Can you work these out from the model? Positions are in its coordinate system, mm. A direction names the side the tool comes from. Give positions to 0.01 mm unless a question says otherwise; leave off trailing zeros. Order: outer loops, then holes, each group sorted by start corner. A loop starts at its lowest first (then second) coordinate and runs counter-clockwise, first axis right, second up. Notation, with made-up numbers: (32.25, 40.25) - (83.25, 40.25) arc R19 ccw to (83.25, 68.25) - close; hole circle Ø9 at (68.5, 79.5). An arc over 180 degrees is marked (long way). Return JSON: item names as keys, results as strings.
```python
from build123d import *

# Parameters (mm, degrees)
SKETCH1_W               = 95.25
SKETCH1_H               = 8.466666667
BOSS_EXTRUDE1_DEPTH     = 38.1
SKETCH2_W               = 6.35
SKETCH2_H               = 127
BOSS_EXTRUDE2_DEPTH     = 38.1
SKETCH3_W               = 88.9
SKETCH3_H               = 8.466666667
BOSS_EXTRUDE3_DEPTH     = 38.1
SKETCH4_R               = 11
CUT_EXTRUDE1_DEPTH      = 149.412147835
SKETCH5_R               = 2.15265
CUT_EXTRUDE2_DEPTH      = 149.412147835
FILLET1_R               = 7.62
BOSS_EXTRUDE4_DEPTH     = 38.1
CUT_EXTRUDE8_REACH      = 172.773
CUT_EXTRUDE8_END_RADIUS = 38.1
FILLET2_R               = 11.688947
FILLET3_R               = 11.688947
FILLET4_R               = 6.35
BOSS_EXTRUDE7_START     = -38.1
BOSS_EXTRUDE7_DEPTH     = 38.1
CUT_EXTRUDE12_DEPTH     = 157.640484095


with BuildPart() as part:
    # Sketch1 → Boss-Extrude1 (new body)
    with BuildSketch(Plane(origin=(0, 0, 0), x_dir=(1, 0, 0), z_dir=(0, 1, 0))):
        with Locations((19.05, 13.758333334)):
            Rectangle(SKETCH1_W, SKETCH1_H)
    extrude(amount=BOSS_EXTRUDE1_DEPTH)

    # Sketch2 → Boss-Extrude2 (add)
    with BuildSketch(Plane(origin=(0, 38.1, 0), x_dir=(1, 0, 0), z_dir=(0, 1, 0))):
        with Locations((63.5, 73.025)):
            Rectangle(SKETCH2_W, SKETCH2_H)
    extrude(amount=-BOSS_EXTRUDE2_DEPTH)

    # Sketch3 → Boss-Extrude3 (add)
    with BuildSketch(Plane(origin=(0, 38.1, 0), x_dir=(1, 0, 0), z_dir=(0, 1, 0))):
        with Locations((15.875, 132.291666667)):
            Rectangle(SKETCH3_W, SKETCH3_H)
    extrude(amount=-BOSS_EXTRUDE3_DEPTH)

    # Sketch4 → Cut-Extrude1 (cut, through all)
    with BuildSketch(Plane(origin=(0, 0, -136.525), x_dir=(-1, 0, 0), z_dir=(0, 0, -1))):
        with Locations((-31.75, 19.05)):
            Circle(SKETCH4_R)
    extrude(amount=-CUT_EXTRUDE1_DEPTH, mode=Mode.SUBTRACT)

    # Sketch5 → Cut-Extrude2 (cut, through all)
    with BuildSketch(Plane(origin=(0, 0, -136.525), x_dir=(-1, 0, 0), z_dir=(0, 0, -1))):
        with Locations((-18.877667779, 26.704865736)):
            Circle(SKETCH5_R)
        with Locations((-19.228536904, 10.833743663)):
            Circle(SKETCH5_R)
        with Locations((-44.622332221, 11.395134264)):
            Circle(SKETCH5_R)
        with Locations((-44.271463096, 27.266256337)):
            Circle(SKETCH5_R)
    extrude(amount=-CUT_EXTRUDE2_DEPTH, mode=Mode.SUBTRACT)

    # Fillet1
    fillet1_edges = [part.edges().sort_by_distance(p)[0] for p in [
        (66.675, 19.05, -136.525),
        (66.675, 19.05, -9.525),
    ]]
    fillet(fillet1_edges, radius=FILLET1_R)

    # Sketch10 → Boss-Extrude4 (add)
    with BuildSketch(Plane(origin=(0, 38.1, 0), x_dir=(1, 0, 0), z_dir=(0, 1, 0))):
        with BuildLine():
            Line((-28.575, 17.991666667), (-28.575, 9.525))
            Line((-28.575, 9.525), (-34.925, 9.525))
            Line((-34.925, 9.525), (-34.925, 25.781))
            Line((-34.925, 25.781), (-5.996027965, 57.15))
            ThreePointArc((-5.996027965, 57.15), (-2.531188929, 73.025), (-5.996027965, 88.9))
            Line((-5.996027965, 88.9), (-34.925, 120.269))
            Line((-34.925, 120.269), (-34.925, 136.525))
            Line((-34.925, 136.525), (-28.575, 136.525))
            Line((-28.575, 136.525), (-28.575, 123.825))
            Line((-28.575, 123.825), (-10.494392478, 104.219375))
            ThreePointArc((-10.494392478, 104.219375), (2.742945437, 73.025), (-10.494392478, 41.830625))
            Line((-10.494392478, 41.830625), (-28.575, 22.225))
            Line((-28.575, 22.225), (-28.575, 17.991666667))
        make_face()
    extrude(amount=-BOSS_EXTRUDE4_DEPTH)

    # Cut-Extrude8: up to this cylinder (the profile starts outside it)
    cut_extrude8_end = Plane(origin=(-40.631188929, 4.042536, -73.025), z_dir=(0, 1, 0)) * Cylinder(CUT_EXTRUDE8_END_RADIUS, 422.746, mode=Mode.PRIVATE)
    # Sketch12 → Cut-Extrude8 (cut, up to the surface)
    with BuildSketch(Plane.ZY.offset(-60.325), mode=Mode.PRIVATE) as cut_extrude8_sk1:
        with BuildLine():
            Line((-82.55, 0), (-63.5, 0))
            ThreePointArc((-63.5, 0), (-73.025, 9.525), (-82.55, 0))
        make_face()
    cut_extrude8_tool1 = extrude(cut_extrude8_sk1.sketch, amount=CUT_EXTRUDE8_REACH, mode=Mode.PRIVATE) - cut_extrude8_end
    add(cut_extrude8_tool1.solids().sort_by_distance((60.325, 4.042536, -73.025))[0], mode=Mode.SUBTRACT)

    # Fillet2
    fillet2_edges = [part.edges().sort_by_distance(p)[0] for p in [
        (-34.925, 19.05, -136.525),
        (-34.925, 19.05, -120.269),
    ]]
    fillet(fillet2_edges, radius=FILLET2_R - 0.0001)  # a hair under: the kernel refuses the full size

    # Fillet3
    fillet3_edges = [part.edges().sort_by_distance(p)[0] for p in [
        (-34.925, 19.05, -25.781),
        (-34.925, 19.05, -9.525),
    ]]
    fillet(fillet3_edges, radius=FILLET3_R - 0.0001)  # a hair under: the kernel refuses the full size

    # Fillet4
    fillet4_edges = [part.edges().sort_by_distance(p)[0] for p in [
        (60.325, 19.05, -17.991666667),
        (60.325, 19.05, -128.058333333),
    ]]
    fillet(fillet4_edges, radius=FILLET4_R)

    # Sketch15 → Boss-Extrude7 (add)
    with BuildSketch(Plane(origin=(0, 38.1, 0), x_dir=(1, 0, 0), z_dir=(0, 1, 0)).offset(BOSS_EXTRUDE7_START)):
        with BuildLine():
            Line((-27.874453006, 23.470813729), (-27.581873113, 23.301892649))
            Line((-27.581873113, 23.301892649), (-25.057662874, 26.039008606))
            ThreePointArc((-25.057662874, 26.039008606), (-34.066608211, 16.896224406), (-21.277878592, 17.991666667))
            Line((-21.277878592, 17.991666667), (-24.699453006, 17.991666667))
            Line((-24.699453006, 17.991666667), (-24.699453006, 17.971552415))
            Line((-24.699453006, 17.971552415), (-27.874453006, 16.13846531))
            Line((-27.874453006, 16.13846531), (-31.049453006, 17.971552415))
            Line((-31.049453006, 17.971552415), (-31.049453006, 21.637726624))
            Line((-31.049453006, 21.637726624), (-27.874453006, 23.470813729))
        make_face()
        with BuildLine():
            Line((-27.581873113, 23.301892649), (-24.699453006, 21.637726624))
            Line((-24.699453006, 21.637726624), (-24.699453006, 17.991666667))
            Line((-24.699453006, 17.991666667), (-21.277878592, 17.991666667))
            ThreePointArc((-21.277878592, 17.991666667), (-21.094704511, 18.889940166), (-21.033278796, 19.804639519))
            ThreePointArc((-21.033278796, 19.804639519), (-22.126765794, 23.514862731), (-25.057662874, 26.039008606))
            Line((-25.057662874, 26.039008606), (-27.581873113, 23.301892649))
        make_face()
        with BuildLine():
            ThreePointArc((60.325, 26.609850645), (54.403432166, 24.225341495), (53.027878592, 17.991666667))
            Line((53.027878592, 17.991666667), (53.975, 17.991666667))
            ThreePointArc((53.975, 17.991666667), (55.237426297, 18.118421545), (56.449453006, 18.493625771))
            Line((56.449453006, 18.493625771), (56.449453006, 21.637726624))
            Line((56.449453006, 21.637726624), (59.624453006, 23.470813729))
            Line((59.624453006, 23.470813729), (60.208975135, 23.13333972))
            ThreePointArc((60.208975135, 23.13333972), (60.295927231, 23.734724375), (60.325, 24.341666667))
            Line((60.325, 24.341666667), (60.325, 26.609850645))
        make_face()
        with BuildLine():
            Line((53.975, 17.991666667), (53.027878592, 17.991666667))
            ThreePointArc((53.027878592, 17.991666667), (60.539152358, 13.024891024), (66.465627215, 19.804639519))
            ThreePointArc((66.465627215, 19.804639519), (64.703538976, 24.387711662), (60.325, 26.609850645))
            Line((60.325, 26.609850645), (60.325, 24.341666667))
            ThreePointArc((60.325, 24.341666667), (60.295927231, 23.734724375), (60.208975135, 23.13333972))
            Line((60.208975135, 23.13333972), (62.799453006, 21.637726624))
            Line((62.799453006, 21.637726624), (62.799453006, 17.971552415))
            Line((62.799453006, 17.971552415), (59.624453006, 16.13846531))
            Line((59.624453006, 16.13846531), (56.449453006, 17.971552415))
            Line((56.449453006, 17.971552415), (56.449453006, 18.493625771))
            ThreePointArc((56.449453006, 18.493625771), (55.237426297, 18.118421545), (53.975, 17.991666667))
        make_face()
        with BuildLine():
            Line((60.325, 121.708333333), (60.325, 119.440149355))
            ThreePointArc((60.325, 119.440149355), (64.703538976, 121.662288338), (66.465627215, 126.245360481))
            ThreePointArc((66.465627215, 126.245360481), (60.539152358, 133.025108976), (53.027878592, 128.058333333))
            Line((53.027878592, 128.058333333), (53.975, 128.058333333))
            ThreePointArc((53.975, 128.058333333), (55.237426297, 127.931578455), (56.449453006, 127.556374229))
            Line((56.449453006, 127.556374229), (56.449453006, 128.078447585))
            Line((56.449453006, 128.078447585), (59.624453006, 129.91153469))
            Line((59.624453006, 129.91153469), (62.799453006, 128.078447585))
            Line((62.799453006, 128.078447585), (62.799453006, 124.412273376))
            Line((62.799453006, 124.412273376), (60.208975135, 122.91666028))
            ThreePointArc((60.208975135, 122.91666028), (60.295927231, 122.315275625), (60.325, 121.708333333))
        make_face()
        with BuildLine():
            ThreePointArc((53.027878592, 128.058333333), (54.403432166, 121.824658505), (60.325, 119.440149355))
            Line((60.325, 119.440149355), (60.325, 121.708333333))
            ThreePointArc((60.325, 121.708333333), (60.295927231, 122.315275625), (60.208975135, 122.91666028))
            Line((60.208975135, 122.91666028), (59.624453006, 122.579186271))
            Line((59.624453006, 122.579186271), (56.449453006, 124.412273376))
            Line((56.449453006, 124.412273376), (56.449453006, 127.556374229))
            ThreePointArc((56.449453006, 127.556374229), (55.237426297, 127.931578455), (53.975, 128.058333333))
            Line((53.975, 128.058333333), (53.027878592, 128.058333333))
        make_face()
        with BuildLine():
            Line((-24.699453006, 128.058333333), (-21.277878592, 128.058333333))
            ThreePointArc((-21.277878592, 128.058333333), (-34.066608211, 129.153775594), (-25.057662874, 120.010991394))
            Line((-25.057662874, 120.010991394), (-27.581873113, 122.748107351))
            Line((-27.581873113, 122.748107351), (-27.874453006, 122.579186271))
            Line((-27.874453006, 122.579186271), (-31.049453006, 124.412273376))
            Line((-31.049453006, 124.412273376), (-31.049453006, 128.078447585))
            Line((-31.049453006, 128.078447585), (-27.874453006, 129.91153469))
            Line((-27.874453006, 129.91153469), (-24.699453006, 128.078447585))
            Line((-24.699453006, 128.078447585), (-24.699453006, 128.058333333))
        make_face()
        with BuildLine():
            ThreePointArc((-21.033278796, 126.245360481), (-21.094704511, 127.160059834), (-21.277878592, 128.058333333))
            Line((-21.277878592, 128.058333333), (-24.699453006, 128.058333333))
            Line((-24.699453006, 128.058333333), (-24.699453006, 124.412273376))
            Line((-24.699453006, 124.412273376), (-27.581873113, 122.748107351))
            Line((-27.581873113, 122.748107351), (-25.057662874, 120.010991394))
            ThreePointArc((-25.057662874, 120.010991394), (-22.126765794, 122.535137269), (-21.033278796, 126.245360481))
        make_face()
    extrude(amount=BOSS_EXTRUDE7_DEPTH)

    # Sketch21 → Cut-Extrude12 (cut, through all)
    with BuildSketch(Plane(origin=(0, 38.1, 0), x_dir=(1, 0, 0), z_dir=(0, 1, 0))):
        Polygon((-24.699453006, 21.637726624), (-27.857033552, 23.460756602), (-31.014614099, 21.637726624), (-31.014614099, 17.991666667), (-27.857033552, 16.168636688), (-24.699453006, 17.991666667), align=None)
        Polygon((56.449453006, 17.991666667), (56.449453006, 21.637726624), (59.607033552, 23.460756602), (62.764614099, 21.637726624), (62.764614099, 17.991666667), (59.607033552, 16.168636688), align=None)
        Polygon((59.607033552, 129.881363312), (56.449453006, 128.058333333), (56.449453006, 124.412273376), (59.607033552, 122.589243398), (62.764614099, 124.412273376), (62.764614099, 128.058333333), align=None)
        Polygon((-24.699453006, 128.058333333), (-24.699453006, 124.412273376), (-27.857033552, 122.589243398), (-31.014614099, 124.412273376), (-31.014614099, 128.058333333), (-27.857033552, 129.881363312), align=None)
    extrude(amount=-CUT_EXTRUDE12_DEPTH, mode=Mode.SUBTRACT)


solid = part.part
```
1. Suppose I cut it at C-C (y = 19.05). State how many separate pieces and enclosed holes the cut face has, plus the area to 3 significant figures.
Checks:
{"separate pieces": "2", "enclosed holes": "4", "area": "2,880 mm^2"}
2. For pin 1 Ø4 at (y, z) = (12.5, -127) entering from -X; pin 2 Ø11.5 at (x, y) = (32.5, 12) entering from -Z (3 decimals); pin 3 Ø2.5 at (x, y) = (18.88, 26.7) entering from -Z, each with a flat end and sliding along its axis, tell me the tip position at first contact or that it passes through.
Checks:
{"pin 1": "x = -34.92", "pin 2": "z = -136.525", "pin 3": "through"}
3. If I drill on L1, parallel to Z at x = 41, y = 8 (3 decimals); L2, parallel to X at y = 31, z = -22 (3 decimals); L3, parallel to Z at x = -28, y = 3, over which ranges is the centre line in solid material (lowest first)? Write a range as [from, to].
Checks:
{"L1": "[-136.525, -128.058], [-17.992, -9.525]", "L2": "[-34.899, -30.387], [-25.327, -21.395], [53.145, 57.077], [62.137, 66.675]", "L3": "[-135.51, -129.8], [-122.67, -112.76], [-33.29, -23.38], [-16.25, -10.54]"}
4. Thinking about a two-plate mould opening in X: for faces 4 (the face through (18, 19, -9.525)), 5 (the face through (-19.09, 19.32, -42.95)), 6 (the face through (60.325, 19, -72)), which applies, +X half, -X half, draft (parallel to the pull), parting line (faces both ways), or undercut?
Checks:
{"face 4": "draft", "face 5": "-X half", "face 6": "undercut"}
5. On a 3-axis mill with a long thin cutter (end or side, diameter ignored), from which of +Z, -Z, +X, -X, +Y, -Y can I reach the whole of each face in a straight line? I mean faces 1 (the face through (-26.3, 19.317, -17.067)), 2 (the face through (-34.146, 18.783, -120.639)), 3 (the face through (17.175, 11.48, -13.818)). Say none if no direction works.
Checks:
{"face 1": "+Y, -Y", "face 2": "-X, +Y, -Y", "face 3": "+Z, -Z"}
6. Suppose I cut it at B-B (x = -17.5). List the corners of the cut face in (y, z) for me (3 decimals), plus the area to 3 significant figures.
Checks:
{"outline": "(0, -136.525) - (38.1, -136.525) - (38.1, -128.058) - (0, -128.058) - close; (0, -111.816) - (38.1, -111.816) - (38.1, -101.374) - (0, -101.374) - close; (0, -44.676) - (38.1, -44.676) - (38.1, -34.234) - (0, -34.234) - close; (0, -17.992) - (38.1, -17.992) - (38.1, -9.525) - (0, -9.525) - close", "area": "1,440 mm^2"}
7. Suppose I cut it at A-A (z = -66.5). List the corners of the cut face in (x, y) for me (3 decimals), plus the area to 3 significant figures.
Checks:
{"outline": "(-3.094, 6.939) - (2.249, 6.939) - (2.249, 38.1) - (-3.094, 38.1) - close; (60.325, 0) - (66.675, 0) - (66.675, 38.1) - (60.325, 38.1) - close", "area": "408 mm^2"}
